from build123d import *

# Parameters (mm, degrees)
BOSS_EXTRUDE1_DEPTH     = 9
SKETCH2_R               = 2.75
BOSS_EXTRUDE2_DEPTH     = 7
CUT_EXTRUDE1_DEPTH      = 33.420493986
CUT_EXTRUDE1_DEPTH_BACK = 33.420493986
FILLET1_R               = 8
FILLET2_R               = 15


with BuildPart() as part:
    # Sketch1 → Boss-Extrude1 (new, symmetric)
    with BuildSketch(Plane.XY):
        with BuildLine():
            Line((-2.5, 9.940447676), (-2.5, 5.728219619))
            ThreePointArc((-2.5, 5.728219619), (0, -6.25), (2.5, 5.728219619))
            Line((2.5, 5.728219619), (2.5, 9.940447676))
            ThreePointArc((2.5, 9.940447676), (0, -10.25), (-2.5, 9.940447676))
        make_face()
    extrude(amount=BOSS_EXTRUDE1_DEPTH, both=True)

    # Sketch2 → Boss-Extrude2 (add, symmetric)
    with BuildSketch(Plane(origin=(0, 0, 0), x_dir=(0, 0, -1), z_dir=(1, 0, 0))):
        with BuildLine():
            Line((-9, 9.940447676), (-7.37704918, 18.792906692))
            ThreePointArc((-7.37704918, 18.792906692), (0, 24.940447676), (7.37704918, 18.792906692))
            Line((7.37704918, 18.792906692), (9, 9.940447676))
            Line((9, 9.940447676), (9, -0.154776162))
            Line((9, -0.154776162), (-9, -0.154776162))
            Line((-9, -0.154776162), (-9, 9.940447676))
        make_face()
        with Locations((0, 17.440447676)):
            Circle(SKETCH2_R, mode=Mode.SUBTRACT)
    extrude(amount=BOSS_EXTRUDE2_DEPTH, both=True)

    # Sketch3 → Cut-Extrude1 (cut, two sides: drawn at the far end of the back side and taken through both)
    with BuildSketch(Plane.XY.offset(9).offset(-CUT_EXTRUDE1_DEPTH_BACK)):
        with BuildLine():
            Line((-2.5, 9.940447676), (-2.5, 24.940447676))
            Line((-2.5, 24.940447676), (2.5, 24.940447676))
            Line((2.5, 24.940447676), (2.5, 9.940447676))
            Line((2.5, 9.940447676), (2.5, 5.728219619))
            ThreePointArc((2.5, 5.728219619), (0, -6.25), (-2.5, 5.728219619))
            Line((-2.5, 5.728219619), (-2.5, 9.940447676))
        make_face()
    extrude(amount=CUT_EXTRUDE1_DEPTH + CUT_EXTRUDE1_DEPTH_BACK, mode=Mode.SUBTRACT)

    # Fillet1
    fillet1_edges = [part.edges().sort_by_distance(p)[0] for p in [
        (-7, 7.487489566, 0),
        (7, 7.487489566, 0),
        (-2.5, 5.728219619, 0),
        (2.5, 5.728219619, 0),
    ]]
    fillet(fillet1_edges, radius=FILLET1_R)

    # Fillet2
    fillet2_edges = [part.edges().sort_by_distance(p)[0] for p in [
        (-4.756470892, 9.940447676, 9),
        (4.756470892, 9.940447676, 9),
        (4.756470892, 9.940447676, -9),
        (-4.756470892, 9.940447676, -9),
    ]]
    fillet(fillet2_edges, radius=FILLET2_R)


solid = part.part
Could you check a few things on this model? Use its own coordinates, in mm. A direction names the side the tool comes from. Round coordinates to 2 decimals unless told otherwise and drop trailing zeros. Order: outer loops, then holes, each group sorted by start corner. A loop starts at its lowest first (then second) coordinate and runs counter-clockwise, first axis right, second up.
(1) Which directions (+Z, -Z, +X, -X, +Y, -Y) give clear straight access to the entire face, cutting with the end or side of a thin tool? Please do faces 1 (the flat face through (0, -7, 9)), 2 (the flat face through (-7, 14.5, -0.1)), 3 (the cylindrical face through (3.06, 6.69, 0.13)).
Response values:
face 1: +Z, +X, -X, +Y, -Y
face 2: +Z, -Z, -X, +Y
face 3: +Z, -Z
(2) Imagine slicing it at D-D (y = -5.5). Write out the boundary of the cut face in (x, z), plus the area to 3 significant figures.
Response values:
outline: (-8.65, -9) - (-2.97, -9) - (-2.97, 9) - (-8.65, 9) - close; (2.97, -9) - (8.65, -9) - (8.65, 9) - (2.97, 9) - close
area: 205 mm2
(3) Please list where these lines run through material, in increasing order: line 1 along X through (y, z) = (10.5, 7.75); line 2 along Y through (x, z) = (5.15, 0); line 3 along X through (y, z) = (0, 2.75).
Response values:
line 1: x = -7 to -2.5, 2.5 to 7
line 2: y = -8.86 to -3.54, 3.54 to 14.69, 20.19 to 24.94
line 3: x = -10.25 to -6.25, 6.25 to 10.25
(4) Imagine slicing it at C-C (x = 3.75). Write out the boundary of the cut face in (y, z).
Response values:
outline: (-9.54, -9) - (-5, -9) - (-5, 9) - (-9.54, 9) - close; (5.34, -9) - (8.58, -9) arc R15 ccw to (11.28, -8.75) - (18.79, -7.38) arc R7.5 ccw to (18.79, 7.38) - (11.28, 8.75) arc R15 ccw to (8.58, 9) - (5.34, 9) - close; hole circle Ø5.5 at (17.44, 0)
(5) Imagine slicing it at B-B (z = 0). Write out the boundary of the cut face in (x, y), plus the area to 3 significant figures.
Response values:
outline: (-8.42, 5.84) arc R10.25 ccw (long way) to (8.42, 5.84) arc R8 cw to (7, 10.4) - (7, 14.69) - (2.5, 14.69) - (2.5, 9.63) arc R8 ccw to (4.61, 4.23) arc R6.25 cw (long way) to (-4.61, 4.23) arc R8 ccw to (-2.5, 9.63) - (-2.5, 14.69) - (-7, 14.69) - (-7, 10.4) arc R8 cw to start; (-7, 20.19) - (-2.5, 20.19) - (-2.5, 24.94) - (-7, 24.94) - close; (2.5, 20.19) - (7, 20.19) - (7, 24.94) - (2.5, 24.94) - close
area: 279 mm2
(6) Imagine slicing it at A-A (y = 0). Write out the boundary of the cut face in (x, z).
Response values:
outline: (-10.25, -9) - (-6.25, -9) - (-6.25, 9) - (-10.25, 9) - close; (6.25, -9) - (10.25, -9) - (10.25, 9) - (6.25, 9) - close
(7) If we mould it in two halves opening along Y, with no side actions, what happens to faces 4 (the cylindrical face through (-3.06, 6.69, 0.13)), 5 (the flat face through (-2.5, 14, 0)), 6 (the cylindrical face through (-4.72, 24.94, 0.15)), 7 (the cylindrical face through (-4.78, 19.76, -1.48))? For each: released by +Y, released by -Y, zero draft, split by the parting line, or undercut.
Response values:
face 4: undercut
face 5: zero draft
face 6: released by +Y
face 7: undercut
(8) I'm going to push flat-ended pins straight in: pin 1 (1 mm diameter, centred on y = 5, z = -1, fed in from +X); pin 2 (10 mm diameter, centred on y = 12, z = 2, fed in from -X); pin 3 (1 mm diameter, centred on x = 4.5, y = 14, fed in from -Z); pin 4 (5 mm diameter, centred on x = -1, y = 6, fed in from -Z). Where does each tip first touch, or does it pass through?
Response values:
pin 1: stops at x = 9.21
pin 2: stops at x = -7.76
pin 3: stops at z = -8.35
pin 4: stops at z = -9
